Part model, mm, in its own coordinate system. A direction names the side the tool comes from. Round coordinates to 2 decimals unless told otherwise and drop trailing zeros. Write each loop counter-clockwise with the first axis right and the second up, starting at its lowest first coordinate (ties: lowest second). Pieces come first, ordered by that corner, then holes.
```python
from build123d import *

# Parameters (mm, degrees)
SKETCH1_W               = 10
SKETCH1_H               = 40
BOSS_EXTRUDE1_DEPTH     = 5
SKETCH2_R               = 2.501304298
SKETCH5_R               = 3
BOSS_EXTRUDE2_DEPTH     = 5
LPATTERN2_COUNT         = 4
LPATTERN2_PITCH         = 10
LPATTERN5_COUNT         = 4
LPATTERN5_PITCH         = 10
CUT_EXTRUDE2_DEPTH      = 33
CUT_EXTRUDE2_DEPTH_BACK = 9
FILLET4_R               = 0.1


with BuildPart() as part:
    # Sketch1 → Boss-Extrude1 (new body)
    with BuildSketch(Plane.XY):
        Rectangle(SKETCH1_W, SKETCH1_H)
    extrude(amount=BOSS_EXTRUDE1_DEPTH)

    # Sweep1: sweep along a path in Sketch3
    with BuildLine(Plane(origin=(0, 0, 0), x_dir=(0, 0, -1), z_dir=(1, 0, 0))) as sweep1_path:
        Line((0, 15), (10, 15))
        ThreePointArc((10, 15), (17.071067812, 12.071067812), (20, 5))
        Line((20, 5), (20, -5))
        ThreePointArc((20, -5), (17.071067812, -12.071067812), (10, -15))
        Line((10, -15), (0, -15))
    # Sketch2 → Sweep1 (sweep)
    with BuildSketch(Plane(origin=(0, 0, 0), x_dir=(-1, 0, 0), z_dir=(0, 0, -1))):
        with Locations((0, 15)):
            Circle(SKETCH2_R)
    sweep(path=sweep1_path.line)

    # Sketch5 → Boss-Extrude2 (add)
    with BuildSketch(Plane.XY.offset(5)):
        with Locations((0, 15)):
            Circle(SKETCH5_R)
    boss_extrude2 = extrude(amount=BOSS_EXTRUDE2_DEPTH)

    # Sketch9 → Revolve2 (revolve)
    with BuildSketch(Plane(origin=(0, 0, 0), x_dir=(0, 0, -1), z_dir=(1, 0, 0))):
        with BuildLine():
            Line((-10, 15), (-14, 15))
            add(Edge.make_bspline(
                [(-10, 18), (-13.224740058, 17.941244514), (-14.000011991, 15.685721652), (-14, 15)],
                knots=[0, 0, 0, 0, 1, 1, 1, 1], degree=3))
            Line((-10, 18), (-10, 15))
        make_face()
    revolve2 = revolve(axis=Axis((0, 15, 10), (0, 0, 1)))

    # LPattern2: Boss-Extrude2 ×4
    with Locations(*[(0, -i * LPATTERN2_PITCH, 0) for i in range(1, LPATTERN2_COUNT)]):
        add(boss_extrude2)

    # LPattern5: Revolve2 ×4
    with Locations(*[(0, -i * LPATTERN5_PITCH, 0) for i in range(1, LPATTERN5_COUNT)]):
        add(revolve2)

    # Sketch12 → Cut-Extrude2 (cut, two sides)
    with BuildSketch(Plane(origin=(0, 12, 0), x_dir=(-1, 0, 0), z_dir=(0, -1, 0))) as cut_extrude2_sk:
        Polygon((-0.766044443, -12.68721239), (-4.506475593, -10.527673459), (-3.542294178, -9.378606794), align=None)
    extrude(amount=CUT_EXTRUDE2_DEPTH, mode=Mode.SUBTRACT)
    extrude(cut_extrude2_sk.sketch, amount=-CUT_EXTRUDE2_DEPTH_BACK, mode=Mode.SUBTRACT)

    # Fillet4
    fillet4_edges = [part.edges().sort_by_distance(p)[0] for p in [
        (0.766044443, 15, 12.68721239),
        (0.766044443, 5, 12.68721239),
        (0.766044443, -5, 12.68721239),
        (0.766044443, -15, 12.68721239),
    ]]
    fillet(fillet4_edges, radius=FILLET4_R)


solid = part.part
```
Q1. Which spindle directions (+Z, -Z, +X, -X, +Y, -Y) get a long thin tool onto all of the face, cutting with end or side? Do faces 5 (the cylindrical face through (0, -2, 7)), 6 (the flat face through (1.836, 14.972, 12.07)), 7 (the cylindrical face through (0.542, -0.07, -17.558)), 8 (the flat face through (0, -20, 2)). Say none if no direction does.
Values follow:
face 5: +Z
face 6: +Y, -Y
face 7: none
face 8: +Z, -Z, +X, -X, -Y
Q2. Cut at C-C on z = 10.5. State how many separate pieces and enclosed holes the cut face has, plus the area to 3 significant figures.
Values follow:
separate pieces: 4
enclosed holes: 0
area: 108 mm2
Q3. Wall check: L1, parallel to Y at x = 0, z = -8; L2, parallel to Y at x = -1.25, z = -3.5; L3, parallel to Y at x = 0.75, z = 6. Give the ranges that are in metal, low to high.
Values follow:
L1: y = -17.5 to -12.5, 12.5 to 17.5
L2: y = -17.17 to -12.83, 12.83 to 17.17
L3: y = -17.9 to -12.1, -7.9 to -2.1, 2.1 to 7.9, 12.1 to 17.9
Q4. Cut at A-A on z = -7. Write the cut outline in (x, y), plus the area to 3 significant figures.
Values follow:
outline: circle Ø5 at (0, -15); circle Ø5 at (0, 15)
area: 39.3 mm2
Q5. Drop flat-ended pins along their axis: pin 1 (6 mm diameter, centred on x = -3, y = -14, fed in from +Z); pin 2 (12 mm diameter, centred on y = 10, z = -19, fed in from +X); pin 3 (3 mm diameter, centred on x = -1.5, y = 3, fed in from +Z). Give the stop position or say it passes through.
Values follow:
pin 1: stops at z = 13.99
pin 2: stops at x = 2.5
pin 3: stops at z = 13.72
Q6. Cut at B-B on x = 3.5. Write the cut outline in (y, z), plus the area to 3 significant figures.
Values follow:
outline: (-20, 0) - (20, 0) - (20, 5) - (-20, 5) - close
area: 200 mm2
Q7. Mould opens along Z. For faces 1 (the flat face through (1.836, -4.972, 12.07)), 2 (the flat face through (0, 0, 5)), 3 (the flat face through (0, 20, 2)), 4 (the flat face through (1.836, 5.028, 12.07)) say: +Z half, -Z half, draft (parallel to the pull), parting line (faces both ways), or undercut.
Values follow:
face 1: undercut
face 2: +Z half
face 3: draft
face 4: undercut
